from build123d import *

# Parameters (mm, degrees)
SKETCH1_W           = 30
SKETCH1_H           = 39
BOSS_EXTRUDE1_DEPTH = 2
SKETCH2_W           = 5
SKETCH2_H           = 39
BOSS_EXTRUDE2_DEPTH = 80
CUT_EXTRUDE1_DEPTH  = 39
SKETCH4_W           = 20
SKETCH4_H           = 39
BOSS_EXTRUDE3_DEPTH = 9
SKETCH5_W           = 5
SKETCH5_H           = 35
CUT_EXTRUDE2_DEPTH  = 30
SKETCH6_W           = 12.5
SKETCH6_H           = 39
CUT_EXTRUDE3_DEPTH  = 2
BOSS_EXTRUDE4_DEPTH = 39
BOSS_EXTRUDE5_DEPTH = 39
SKETCH10_W          = 5
SKETCH10_H          = 35
CUT_EXTRUDE4_DEPTH  = 10


with BuildPart() as part:
    # Sketch1 → Boss-Extrude1 (new body)
    with BuildSketch(Plane.XY):
        Rectangle(SKETCH1_W, SKETCH1_H)
    extrude(amount=BOSS_EXTRUDE1_DEPTH)

    # Sketch2 → Boss-Extrude2 (add)
    with BuildSketch(Plane.XY.offset(2)):
        Rectangle(SKETCH2_W, SKETCH2_H)
    extrude(amount=BOSS_EXTRUDE2_DEPTH)

    # Sketch3 → Cut-Extrude1 (cut)
    with BuildSketch(Plane.XZ.offset(19.5)):
        Polygon((-2.5, 82), (2.5, 82), (2.5, 77), align=None)
    extrude(amount=-CUT_EXTRUDE1_DEPTH, mode=Mode.SUBTRACT)

    # Sketch4 → Boss-Extrude3 (add)
    with BuildSketch(Plane(origin=(39.75, 0, 39.75), x_dir=(0.707106781, 0, -0.707106781), z_dir=(0.707106781, 0, 0.707106781))):
        with Locations((-49.75052301, 0)):
            Rectangle(SKETCH4_W, SKETCH4_H)
    extrude(amount=BOSS_EXTRUDE3_DEPTH)

    # Sketch5 → Cut-Extrude2 (cut)
    with BuildSketch(Plane(origin=(-28.107864376, 0, 28.107864376), x_dir=(-0.707106781, 0, -0.707106781), z_dir=(0.707106781, 0, -0.707106781))):
        with Locations((-60.714989104, 0)):
            Rectangle(SKETCH5_W, SKETCH5_H)
    extrude(amount=-CUT_EXTRUDE2_DEPTH, mode=Mode.SUBTRACT)

    # Sketch6 → Cut-Extrude3 (cut)
    with BuildSketch(Plane.XY.offset(2)):
        with Locations((-8.75, 0)):
            Rectangle(SKETCH6_W, SKETCH6_H)
    extrude(amount=-CUT_EXTRUDE3_DEPTH, mode=Mode.SUBTRACT)

    # Sketch7 → Boss-Extrude4 (add)
    with BuildSketch(Plane.XZ.offset(19.5)):
        Polygon((-2.5, 82), (3.863961031, 88.363961031), (-2.5, 88.363961031), align=None)
    extrude(amount=-BOSS_EXTRUDE4_DEPTH)

    # Sketch8 → Boss-Extrude5 (add)
    with BuildSketch(Plane.XZ.offset(19.5)):
        Polygon((2.5, 77), (11.642135624, 67.857864376), (2.5, 67.857864376), align=None)
    extrude(amount=-BOSS_EXTRUDE5_DEPTH)

    # Sketch10 → Cut-Extrude4 (cut)
    with BuildSketch(Plane(origin=(-42.25, 0, 42.25), x_dir=(-0.707106781, 0, -0.707106781), z_dir=(0.707106781, 0, -0.707106781))):
        with Locations((-60.714989104, 0)):
            Rectangle(SKETCH10_W, SKETCH10_H)
    extrude(amount=-CUT_EXTRUDE4_DEPTH, mode=Mode.SUBTRACT)


solid = part.part
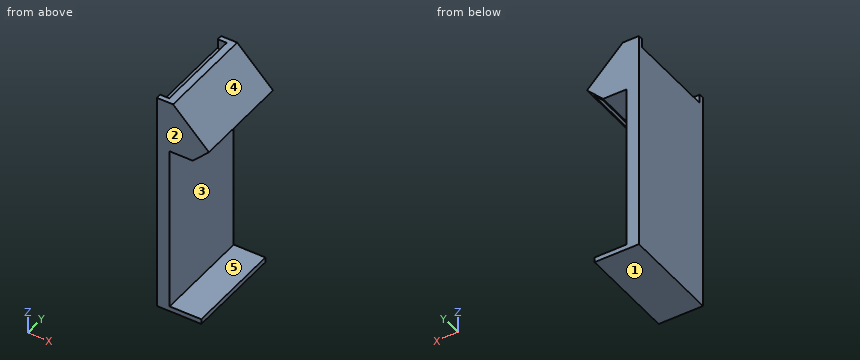
Design review of the part built by this model. Coordinates are the model's own, in mm. Face numbers are marked on the shaded views. A direction names the side the tool comes from. Coordinates: 2 decimals unless noted, no trailing zeros. Loops run counter-clockwise (first coordinate to the right, second up) from the corner with the lowest first, then second, coordinate; pieces in that order, holes last. Notation, with made-up numbers: M 28.5,-29 L 87.5,-29 A10 cw 87.5,-11 Z; hole C 5,83 d9. An arc over 180 degrees is marked long. Answer as CSV lines item,"result".
Item 1: For P1, Ø1, axis at y = -13.5, z = 17, coming from the +X side; P2, Ø1, axis at y = -9, z = 1, coming from the +X side, all flat-tipped, find the tip position at first contact; note any pin that passes through.
Answer list:
P1,"x = 2.5"
P2,"x = 15"
Item 2: For probe 1 along Z at (x, y) = (3.25, 6); probe 2 along Y at (x, z) = (7, 80); probe 3 along Z at (x, y) = (5, -13.5), list the stretches that pass through material, from the lowest coordinate up.
Answer list:
probe 1,"0 to 2, 67.86 to 79.08, 86.15 to 88.36"
probe 2,"-19.5 to -17.5, 17.5 to 19.5"
probe 3,"0 to 2, 67.86 to 77.33, 84.4 to 87.23"
Item 3: Add section C-C on z = 78. State the section outline as (x, y) points, plus the area to 3 significant figures.
Answer list:
outline,"M -2.5,-19.5 L 14.23,-19.5 L 14.23,19.5 L -2.5,19.5 Z; hole M 4.33,-17.5 L 11.4,-17.5 L 11.4,17.5 L 4.33,17.5 Z"
area,"405 mm²"
Item 4: Add section B-B on y = 0. State the section outline as (x, z) points, plus the area to 3 significant figures.
Answer list:
outline,"M -2.5,0 L 15,0 L 15,2 L 2.5,2 L 2.5,67.86 L 11.64,67.86 L 13.06,69.27 L -2.5,84.83 Z; M 1.04,88.36 L 16.59,72.81 L 18.01,74.22 L 3.86,88.36 Z"
area,"548 mm²"
Item 5: The part is to be moulded in two halves that separate along Z. For the marked faces 1, 2 and 3, say which applies: pulls with the +Z half, pulls with the -Z half, needs draft (parallel to the pull), parting line crosses it, or undercut.
Answer list:
face 1,"pulls with the -Z half"
face 2,"needs draft"
face 3,"undercut"
Item 6: Add section D-D on x = 6. State the section outline as (y, z) points, plus the area to 3 significant figures.
Answer list:
outline,"M -19.5,0 L 19.5,0 L 19.5,2 L -19.5,2 Z; M -19.5,67.86 L 19.5,67.86 L 19.5,86.23 L -19.5,86.23 Z; hole M -17.5,76.33 L 17.5,76.33 L 17.5,83.4 L -17.5,83.4 Z"
area,"547 mm²"
Item 7: Add section A-A on x = 10.25. State the section outline as (y, z) points.
Answer list:
outline,"M -19.5,0 L 19.5,0 L 19.5,2 L -19.5,2 Z; M -19.5,67.86 L 19.5,67.86 L 19.5,81.98 L -19.5,81.98 Z; hole M -17.5,72.08 L 17.5,72.08 L 17.5,79.15 L -17.5,79.15 Z"
Item 8: Machinability: for the marked faces 4 and 5, which of the approach directions +Z, -Z, +X, -X, +Y, -Y give a long, thin tool a straight path to every point of the face, cutting with its end or side? Answer none if there is none.
Answer list:
face 4,"+Z, +X, +Y, -Y"
face 5,"+X, +Y, -Y"
